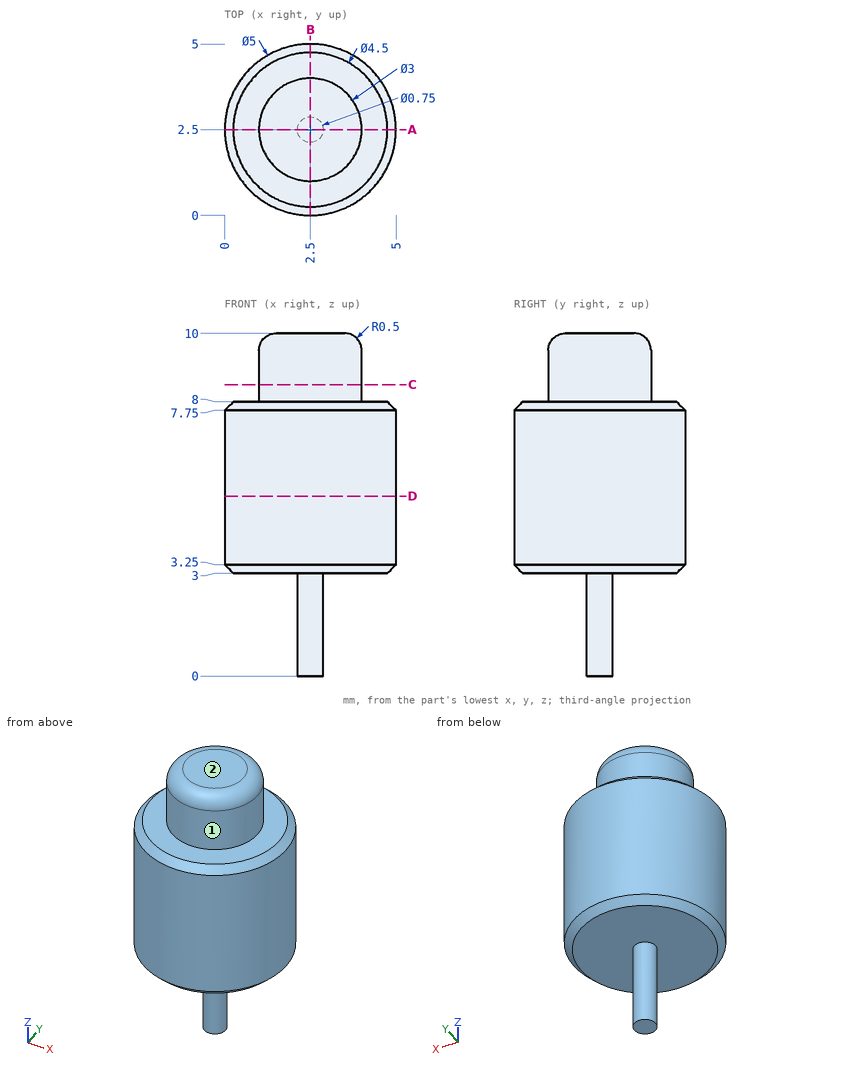
Could you check a few things on this drawing? It's one solid part, dimensions in mm from its lowest x, y, z. A direction names the side the tool comes from. Coordinates: 2 decimals unless noted, no trailing zeros. Loops run counter-clockwise (first coordinate to the right, second up) from the corner with the lowest first, then second, coordinate; pieces in that order, holes last. Notation, with made-up numbers: (-22.75, 34) - (-17.75, 34) arc R11 cw to (-17.75, 53) - close; hole circle Ø6 at (20.25, -40). An arc over 180 degrees is marked (long way). Answer as a JSON object with one key per item and string values. Group by question number.
Item 1: For pin 1 (1 mm diameter, centred on y = 1.5, z = 7.5, fed in from -X); pin 2 (2 mm diameter, centred on x = 1.5, y = 4, fed in from -Z), each with a flat end and sliding along its axis, tell me the tip position at first contact or that it passes through.
Item 2: If we section it at A-A (y = 2.5): List the corners of the cut face in (x, z) for me (3 decimals), plus the area to 3 significant figures.
Item 3: On a 3-axis mill with a long thin cutter (end or side, diameter ignored), from which of +Z, -Z, +X, -X, +Y, -Y can I reach the whole of each face in a straight line? I mean the marked faces 1 and 2. Say none if no direction works.
Item 4: If I drill on L1, parallel to Z at x = 3, y = 2.7; L2, parallel to Z at x = 3.75, y = 1; L3, parallel to Y at x = 2.5, z = 1.5 (3 decimals), over which ranges is the centre line in solid material (lowest first)? Write a range as from..to.
Item 5: If we section it at C-C (z = 8.5): List the corners of the cut face in (x, y) for me.
Item 6: If we section it at D-D (z = 5.25): List the corners of the cut face in (x, y) for me.
Returned:
{
 "1": {"pin 1": "stops at x = 0.05", "pin 2": "stops at z = 3"},
 "2": {"outline": "(0, 3.25) - (0.25, 3) - (2.125, 3) - (2.125, 0) - (2.875, 0) - (2.875, 3) - (4.75, 3) - (5, 3.25) - (5, 7.75) - (4.75, 8) - (4, 8) - (4, 9.5) arc R0.5 ccw to (3.5, 10) - (1.5, 10) arc R0.5 ccw to (1, 9.5) - (1, 8) - (0.25, 8) - (0, 7.75) - close", "area": "33.0 mm²"},
 "3": {"face 1": "+Z", "face 2": "+Z, +X, -X, +Y, -Y"},
 "4": {"L1": "z = 3..10", "L2": "z = 3..8", "L3": "y = 2.125..2.875"},
 "5": {"outline": "circle Ø3 at (2.5, 2.5)"},
 "6": {"outline": "circle Ø5 at (2.5, 2.5)"}
}
